from build123d import *

# Parameters (mm, degrees)
F1_DEPTH = 12
F2_R     = 30
F3_R     = 15


with BuildPart() as f1:
    # F0 (on Top) → F1 (new body)
    with BuildSketch(Plane.XY):
        Polygon((39.4856995648, 193), (37.7842070275, 181), (137.5, 181), (237.2157929725, 181), (235.5143004352, 193), (137.5, 193), align=None)
        Polygon((27.3656716418, 193), (25.6641791045, 181), (37.7842070275, 181), (39.4856995648, 193), align=None)
        Polygon((25.6641791045, 181), (19.9925373134, 141), (32.1125652364, 141), (37.7842070275, 181), align=None)
        Polygon((19.9925373134, 141), (18.2910447761, 129), (30.4110726991, 129), (32.1125652364, 141), align=None)
        Polygon((237.2157929725, 181), (242.8874347636, 141), (255.0074626866, 141), (249.3358208955, 181), align=None)
        Polygon((235.5143004352, 193), (237.2157929725, 181), (249.3358208955, 181), (247.6343283582, 193), align=None)
        Polygon((242.8874347636, 141), (244.5889273009, 129), (256.7089552239, 129), (255.0074626866, 141), align=None)
        Polygon((244.5889273009, 129), (251.6784795397, 79), (263.7985074627, 79), (256.7089552239, 129), align=None)
        Polygon((251.6784795397, 79), (253.379972077, 67), (265.5, 67), (263.7985074627, 79), align=None)
        Polygon((23.3215204603, 79), (21.620027923, 67), (137.5, 67), (253.379972077, 67), (251.6784795397, 79), (137.5, 79), align=None)
        Polygon((253.379972077, 67), (261.1784795397, 12), (273.2985074627, 12), (265.5, 67), align=None)
        Polygon((261.1784795397, 12), (262.879972077, 0), (275, 0), (273.2985074627, 12), align=None)
        Polygon((13.8215204603, 12), (12.120027923, 0), (262.879972077, 0), (261.1784795397, 12), (137.5, 12), align=None)
        Polygon((1.7014925373, 12), (0, 0), (12.120027923, 0), (13.8215204603, 12), align=None)
        Polygon((9.5, 67), (1.7014925373, 12), (13.8215204603, 12), (21.620027923, 67), align=None)
        Polygon((11.2014925373, 79), (9.5, 67), (21.620027923, 67), (23.3215204603, 79), align=None)
        Polygon((18.2910447761, 129), (11.2014925373, 79), (23.3215204603, 79), (30.4110726991, 129), align=None)
        Polygon((32.1125652364, 141), (30.4110726991, 129), (137.5, 129), (244.5889273009, 129), (242.8874347636, 141), (137.5, 141), align=None)
    extrude(amount=F1_DEPTH)

    # F2
    f2_edges = [f1.edges().sort_by_distance(p)[0] for p in [
        (27.365672, 193, 6),
        (247.634328, 193, 6),
    ]]
    fillet(f2_edges, radius=F2_R)

    # F3
    f3_edges = [f1.edges().sort_by_distance(p)[0] for p in [
        (37.784207, 181, 6),
        (237.215793, 181, 6),
    ]]
    fillet(f3_edges, radius=F3_R)


solid = f1.part
The model under review builds one solid part; all positions refer to its coordinate system, in mm. A direction names the side the tool comes from. Round coordinates to 2 decimals unless told otherwise and drop trailing zeros. Loops run counter-clockwise (first coordinate to the right, second up) from the corner with the lowest first, then second, coordinate; pieces in that order, holes last. Notation, with made-up numbers: (25, 66.5) -> (72, 66.5) arc R17 cw to (72, 79.5) -> close; hole circle Ø7 at (68.25, -2). An arc over 180 degrees is marked (long way). One line per question, with ' | ' between items. Start each with the question number.
Item 1: Add section C-C, the plane z = 4.25. Count the separate pieces of the cut face and the enclosed holes in it, then the cut area to 3 significant figures.
Item 2: Add section B-B, the plane y = 104.5. Write out the cut boundary in (x, z), then the cut area to 3 significant figures.
Item 3: Machinability: for faces 1 (the face through (139, 141, 6)), 2 (the face through (137, 133, 0)), which of the approach directions +Z, -Z, +X, -X, +Y, -Y give a long, thin tool a straight path to every point of the face, cutting with its end or side? Answer none if there is none.
Item 4: Draft analysis for pull direction Y (two halves, no side actions). For faces 3 (the face through (248.084, 104.35, 5.916)), 4 (the face through (137, 133, 12)), 5 (the face through (136, 0, 6)), state which applies: +Y half, -Y half, draft (parallel to the pull), parting line (faces both ways), or undercut.
Item 5: Wall thickness on line 1 along Y through (x, z) = (146.5, 2.5); line 2 along Y through (x, z) = (48, 0.5); line 3 along X through (y, z) = (100, 7.5): over which ranges is each line inside the solid? List them lowest first. Write a range as [from, to].
Item 6: For pin 1 (2 mm diameter, centred on y = 101, z = 6.5, fed in from -X); pin 2 (1.5 mm diameter, centred on y = 160.5, z = 1.5, fed in from +X); pin 3 (6 mm diameter, centred on x = 37.5, z = 5, fed in from -Y); pin 4 (5 mm diameter, centred on y = 141.5, z = 10.5, fed in from -X), all flat-tipped, find the tip position at first contact; note any pin that passes through.
Item 7: Add section D-D, the plane y = 134.5. Write out the cut boundary in (x, z), then the cut area to 3 significant figures.
Item 8: Add section A-A, the plane x = 114.5. Write out the cut boundary in (y, z).
Return value:
1) separate pieces: 1 | enclosed holes: 3 | area: 15,100 mm2
2) outline: (14.82, 0) -> (26.94, 0) -> (26.94, 12) -> (14.82, 12) -> close; (248.06, 0) -> (260.18, 0) -> (260.18, 12) -> (248.06, 12) -> close | area: 291 mm2
3) face 1: +Z, -Z | face 2: -Z, +X, -X, +Y, -Y
4) face 3: undercut | face 4: draft | face 5: -Y half
5) line 1: y = [0, 12], [67, 79], [129, 141], [181, 193] | line 2: y = [0, 12], [67, 79], [129, 141], [180.73, 192.51] | line 3: x = [14.18, 26.3], [248.7, 260.82]
6) pin 1: stops at x = 14.18 | pin 2: stops at x = 252.35 | pin 3: stops at y = 0 | pin 4: stops at x = 19.71
7) outline: (19.07, 0) -> (255.93, 0) -> (255.93, 12) -> (19.07, 12) -> close | area: 2,840 mm2
8) outline: (0, 0) -> (12, 0) -> (12, 12) -> (0, 12) -> close; (67, 0) -> (79, 0) -> (79, 12) -> (67, 12) -> close; (129, 0) -> (141, 0) -> (141, 12) -> (129, 12) -> close; (181, 0) -> (193, 0) -> (193, 12) -> (181, 12) -> close
